Job drawing, mm, ordinate dimensions from the low corner. One solid piece. Give positions to 0.01 mm unless a question says otherwise; leave off trailing zeros. Loops run counter-clockwise (first coordinate to the right, second up) from the corner with the lowest first, then second, coordinate; pieces in that order, holes last. Notation, with made-up numbers: (42, -1) - (82, -1) arc R36 cw to (82, 38) - close; hole circle Ø9 at (60.5, 55). An arc over 180 degrees is marked (long way). Use a Markdown table: item, result.
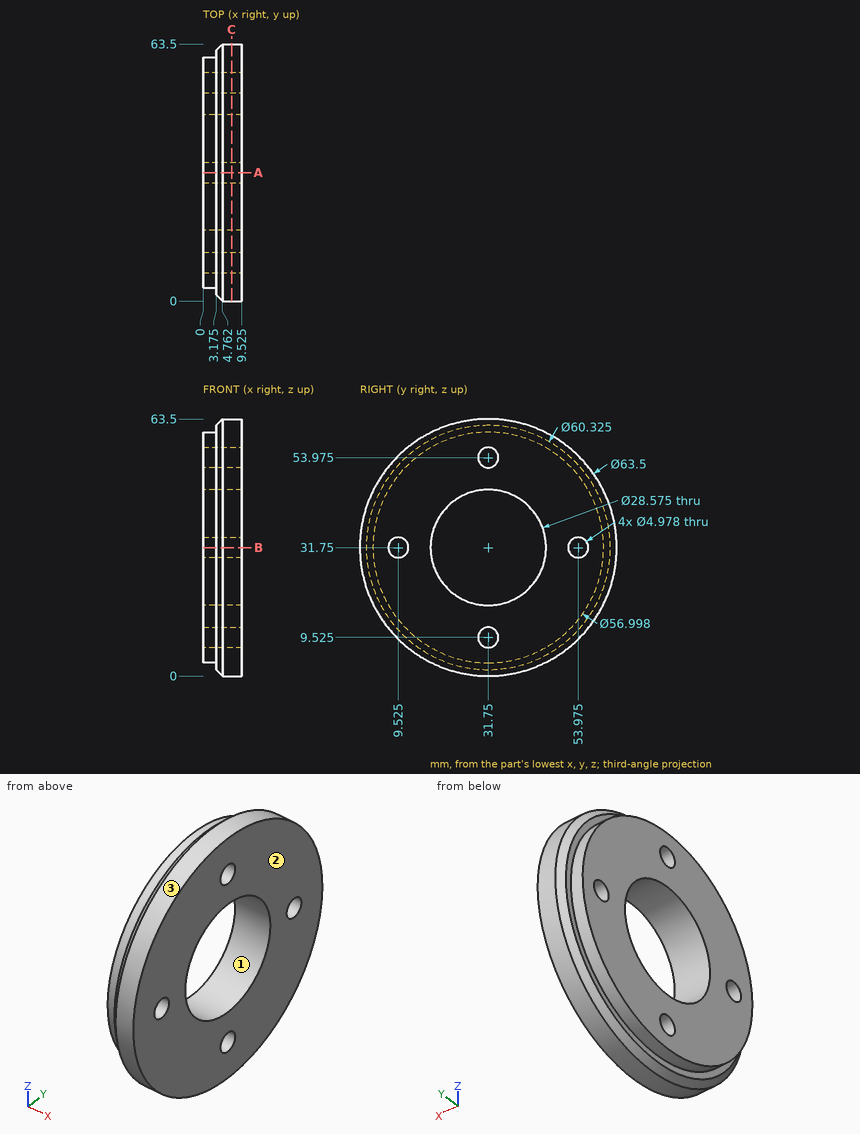
(1) Slice it at C-C, the plane x = 7. Count the separate pieces of the cut face and the enclosed holes in it, plus the area to 3 significant figures.
Computed:
| item | result |
|---|---|
| separate pieces | 1 |
| enclosed holes | 5 |
| area | 2,450 mm² |
(2) Slice it at A-A, the plane y = 31.75. Write the cut outline in (x, z) (1 decimal), plus the area to 3 significant figures.
Computed:
| item | result |
|---|---|
| outline | (0, 3.3) - (3.2, 3.3) - (3.2, 1.6) - (4.8, 0) - (9.5, 0) - (9.5, 7) - (0, 7) - close; (0, 12) - (9.5, 12) - (9.5, 17.5) - (0, 17.5) - close; (0, 46) - (9.5, 46) - (9.5, 51.5) - (0, 51.5) - close; (0, 56.5) - (9.5, 56.5) - (9.5, 63.5) - (4.8, 63.5) - (3.2, 61.9) - (3.2, 60.2) - (0, 60.2) - close |
| area | 215 mm² |
(3) Mould opens along Z. For the marked faces 1, 2 and 3 say: pulls with the +Z half, pulls with the -Z half, needs draft (parallel to the pull), parting line crosses it, or undercut.
Computed:
| item | result |
|---|---|
| face 1 | undercut |
| face 2 | needs draft |
| face 3 | parting line crosses it |
(4) Drill centre lines: probe 1 along Z at (x, y) = (5.5, 31.5) (1 decimal); probe 2 along Y at (x, z) = (2.75, 31.75) (1 decimal); probe 3 along Y at (x, z) = (8.5, 23.5) (1 decimal). Where is each one in solid material? Low to high. Write a range as [from, to].
Computed:
| item | result |
|---|---|
| probe 1 | [0, 7], [12, 17.5], [46, 51.5], [56.5, 63.5] |
| probe 2 | [3.3, 7], [12, 17.5], [46, 51.5], [56.5, 60.2] |
| probe 3 | [1.1, 20.1], [43.4, 62.4] |
(5) Pin check, flat tips, straight feed: P1, Ø5, axis at x = 2.5, z = 28.5, coming from the +Y side (1 decimal); P2, Ø5, axis at x = 3.5, z = 9.5, coming from the +Y side (1 decimal); P3, Ø1, axis at x = 6, y = 24.5, coming from the +Z side (1 decimal). Stop position of each tip, or through.
Computed:
| item | result |
|---|---|
| P1 | y = 63.4 |
| P2 | y = 56.3 |
| P3 | z = 62.8 |
